Geometry check sheet. Reference: the model listing, model coordinates, mm. A direction names the side the tool comes from. Give positions to 0.01 mm unless a question says otherwise; leave off trailing zeros. Order: outer loops, then holes, each group sorted by start corner. A loop starts at its lowest first (then second) coordinate and runs counter-clockwise, first axis right, second up.
from build123d import *

# Parameters (mm, degrees)
SKETCH1_W           = 130
SKETCH1_H           = 64
SKETCH1_R           = 2.9575
BOSS_EXTRUDE1_DEPTH = 10
SKETCH2_W           = 130
SKETCH2_H           = 16
SKETCH2_R           = 2.75
BOSS_EXTRUDE2_DEPTH = 10
SKETCH3_W           = 160
SKETCH3_H           = 70
SKETCH3_R           = 2.25
SKETCH3_R_2         = 5.25
BOSS_EXTRUDE3_DEPTH = 7
SKETCH4_R           = 12
CUT_EXTRUDE1_DEPTH  = 3
FILLET1_R           = 5
CUT_EXTRUDE2_REACH  = 126.282
SKETCH5_R           = 2.9575
FILLET2_R           = 5
FILLET3_R           = 5


with BuildPart() as part:
    # Sketch1 → Boss-Extrude1 (new body)
    with BuildSketch(Plane.XY):
        Rectangle(SKETCH1_W, SKETCH1_H)
        with Locations((57, 16)):
            Circle(SKETCH1_R, mode=Mode.SUBTRACT)
        with Locations((57, -16)):
            Circle(SKETCH1_R, mode=Mode.SUBTRACT)
        with Locations((-57, -16)):
            Circle(SKETCH1_R, mode=Mode.SUBTRACT)
        with Locations((-57, 16)):
            Circle(SKETCH1_R, mode=Mode.SUBTRACT)
    extrude(amount=BOSS_EXTRUDE1_DEPTH)

    # Sketch2 → Boss-Extrude2 (add)
    with BuildSketch(Plane.XZ.offset(32)):
        with Locations((0, -8)):
            Rectangle(SKETCH2_W, SKETCH2_H)
        with Locations(Location((-40, -9, 0), (0, 0, 270))):
            Circle(SKETCH2_R, mode=Mode.SUBTRACT)
        with Locations(Location((40, -9, 0), (0, 0, 90))):
            Circle(SKETCH2_R, mode=Mode.SUBTRACT)
    extrude(amount=-BOSS_EXTRUDE2_DEPTH)

    # Sketch3 → Boss-Extrude3 (add)
    with BuildSketch(Plane(origin=(0, 32, 0), x_dir=(1, 0, 0), z_dir=(0, 1, 0))):
        with Locations((-15, -35)):
            Rectangle(SKETCH3_W, SKETCH3_H)
        with Locations(Location((48, -12.95, 0), (0, 0, 270))):
            Circle(SKETCH3_R, mode=Mode.SUBTRACT)
        with Locations(Location((-4.1, -18.05, 0), (0, 0, 270))):
            Circle(SKETCH3_R, mode=Mode.SUBTRACT)
        with Locations(Location((-4.1, -45.95, 0), (0, 0, 270))):
            Circle(SKETCH3_R, mode=Mode.SUBTRACT)
        with Locations(Location((46.7, -61.15, 0), (0, 0, 270))):
            Circle(SKETCH3_R, mode=Mode.SUBTRACT)
        with Locations(Location((-80, -58, 0), (0, 0, 270))):
            Circle(SKETCH3_R_2, mode=Mode.SUBTRACT)
        with BuildLine():
            Line((-83.039736831, -30.6), (-76.960263169, -30.6))
            ThreePointArc((-76.960263169, -30.6), (-72, -38), (-76.960263169, -45.4))
            Line((-76.960263169, -45.4), (-83.039736831, -45.4))
            ThreePointArc((-83.039736831, -45.4), (-88, -38), (-83.039736831, -30.6))
        make_face(mode=Mode.SUBTRACT)
        with BuildLine():
            Line((-83.039736831, -7.6), (-76.960263169, -7.6))
            ThreePointArc((-76.960263169, -7.6), (-72, -15), (-76.960263169, -22.4))
            Line((-76.960263169, -22.4), (-83.039736831, -22.4))
            ThreePointArc((-83.039736831, -22.4), (-88, -15), (-83.039736831, -7.6))
        make_face(mode=Mode.SUBTRACT)
    extrude(amount=BOSS_EXTRUDE3_DEPTH)

    # Sketch4 → Cut-Extrude1 (cut)
    # profile 1 of 6: a face of its own
    with BuildSketch(Plane.XZ.offset(-32)):
        with Locations((-80, 38)):
            Circle(SKETCH4_R)
    # profile 2 of 6: a face of its own
    with BuildSketch(Plane.XZ.offset(-32)):
        with Locations((-80, 15)):
            Circle(SKETCH4_R)
        with BuildLine():
            Line((-76.960263169, 7.6), (-83.039736831, 7.6))
            ThreePointArc((-83.039736831, 7.6), (-88, 15), (-83.039736831, 22.4))
            Line((-83.039736831, 22.4), (-76.960263169, 22.4))
            ThreePointArc((-76.960263169, 22.4), (-72, 15), (-76.960263169, 7.6))
        make_face(mode=Mode.SUBTRACT)
    # profile 3 of 6: a face of its own
    with BuildSketch(Plane.XZ.offset(-32)):
        with Locations((-80, 15)):
            Circle(SKETCH4_R)
    # profile 4 of 6: a face of its own
    with BuildSketch(Plane.XZ.offset(-32)):
        with Locations((-80, 38)):
            Circle(SKETCH4_R)
        with BuildLine():
            Line((-76.960263169, 30.6), (-83.039736831, 30.6))
            ThreePointArc((-83.039736831, 30.6), (-88, 38), (-83.039736831, 45.4))
            Line((-83.039736831, 45.4), (-76.960263169, 45.4))
            ThreePointArc((-76.960263169, 45.4), (-72, 38), (-76.960263169, 30.6))
        make_face(mode=Mode.SUBTRACT)
    # profile 5 of 6: a face of its own
    with BuildSketch(Plane.XZ.offset(-32)):
        with Locations((-80, 38)):
            Circle(SKETCH4_R)
    # profile 6 of 6: a face of its own
    with BuildSketch(Plane.XZ.offset(-32)):
        with Locations((-80, 15)):
            Circle(SKETCH4_R)
    extrude(amount=-CUT_EXTRUDE1_DEPTH, mode=Mode.SUBTRACT)

    # Fillet1
    fillet1_edges = [part.edges().sort_by_distance(p)[0] for p in [
        (-83.4278273, 33.5, 26.5),
        (-76.5721727, 33.5, 26.5),
    ]]
    fillet(fillet1_edges, radius=FILLET1_R)

    # Sketch5 → Cut-Extrude2 (cut, up to next)
    with BuildSketch(Plane(origin=(0, 0, 0), x_dir=(-1, 0, 0), z_dir=(0, 0, -1)), mode=Mode.PRIVATE) as cut_extrude2_sk1:
        with Locations((-50, -2)):
            Circle(SKETCH5_R)
    cut_extrude2_tool1 = extrude(cut_extrude2_sk1.sketch, amount=-CUT_EXTRUDE2_REACH, mode=Mode.PRIVATE) & part.part
    # Sketch5 → Cut-Extrude2 (cut, up to next)
    with BuildSketch(Plane(origin=(0, 0, 0), x_dir=(-1, 0, 0), z_dir=(0, 0, -1)), mode=Mode.PRIVATE) as cut_extrude2_sk2:
        with Locations((50, -2)):
            Circle(SKETCH5_R)
    cut_extrude2_tool2 = extrude(cut_extrude2_sk2.sketch, amount=-CUT_EXTRUDE2_REACH, mode=Mode.PRIVATE) & part.part
    add(cut_extrude2_tool1.solids().sort_by_distance((50, -2, 0))[0], mode=Mode.SUBTRACT)
    add(cut_extrude2_tool2.solids().sort_by_distance((-50, -2, 0))[0], mode=Mode.SUBTRACT)

    # Fillet2
    fillet2_edges = [part.edges().sort_by_distance(p)[0] for p in [
        (-65, -27, -16),
    ]]
    fillet(fillet2_edges, radius=FILLET2_R)

    # Fillet3
    fillet3_edges = [part.edges().sort_by_distance(p)[0] for p in [
        (65, -27, -16),
    ]]
    fillet(fillet3_edges, radius=FILLET3_R)


solid = part.part
Item 1: Draft check along Y on faces 6 (the flat face through (-16, 32, 42)), 7 (the cylindrical face through (-79.769, 35.451, 52.755)), 8 (the cylindrical face through (-55.41, -13.506, 4.93)). Enter one of: released by +Y, released by -Y, zero draft, split by the parting line, or undercut.
Reported:
face 6: released by -Y
face 7: zero draft
face 8: undercut
Item 2: Sectioned sample at D-D (z = 38). Enter the section's corners in (x, y).
Reported:
outline: (-95, 32) - (-92, 32) - (-92, 35) - (-88, 35) - (-88, 39) - (-95, 39) - close; (-72, 35) - (-68, 35) - (-68, 32) - (65, 32) - (65, 39) - (-72, 39) - close
Item 3: Sectioned sample at C-C (y = -16). Enter the section's corners in (x, z).
Reported:
outline: (-65, 0) - (-59.96, 0) - (-59.96, 10) - (-65, 10) - close; (-54.04, 0) - (54.04, 0) - (54.04, 10) - (-54.04, 10) - close; (59.96, 0) - (65, 0) - (65, 10) - (59.96, 10) - close
Item 4: Gauge pin test, flat ends, axial feed: pin 1 (10 mm diameter, centred on x = -32, z = 52.5, fed in from -Y); pin 2 (3 mm diameter, centred on x = -79, y = 37, fed in from -Z); pin 3 (7 mm diameter, centred on x = 57, y = 16, fed in from +Z). Record the tip position at first contact, or that the pin passes through.
Reported:
pin 1: stops at y = 32
pin 2: stops at z = 0
pin 3: stops at z = 10
Item 5: Sectioned sample at B-B (x = -4.1). Enter the section's corners in (y, z), and give its area (3 significant figures).
Reported:
outline: (-32, -16) - (-22, -16) - (-22, 0) - (39, 0) - (39, 15.8) - (32, 15.8) - (32, 10) - (-32, 10) - close; (32, 20.3) - (39, 20.3) - (39, 43.7) - (32, 43.7) - close; (32, 48.2) - (39, 48.2) - (39, 70) - (32, 70) - close
area: 1,230 mm2
Item 6: Sectioned sample at A-A (z = 61.15). Enter the section's corners in (x, y), and give its area (3 significant figures).
Reported:
outline: (-95, 32) - (-84.2, 32) - (-84.2, 39) - (-95, 39) - close; (-75.8, 32) - (44.45, 32) - (44.45, 39) - (-75.8, 39) - close; (48.95, 32) - (65, 32) - (65, 39) - (48.95, 39) - close
area: 1,030 mm2
Item 7: Scan lines: L1, parallel to X at y = -27.75, z = -9; L2, parallel to Z at x = 40, y = -27; L3, parallel to Y at x = -57, z = 4. Record each from-to range of solid material in increasing order.
Reported:
L1: x = -65 to -42.75, -37.25 to 37.25, 42.75 to 65
L2: z = -16 to -11.75, -6.25 to 10
L3: y = -32 to -18.96, -13.04 to 13.04, 18.96 to 39
Item 8: Set-up check for faces 1 (the flat face through (65, 11, 9)), 2 (the flat face through (-1, -32, -3)), 3 (the cylindrical face through (-80, 33, 3)), 4 (the flat face through (-1, 0, 10)), 5 (the flat face through (-80, 37, 30.6)): record each of +Z, -Z, +X, -X, +Y, -Y from which the full face is reachable in a straight line by a thin tool's end or side.
Reported:
face 1: +Z, -Z, +X, +Y, -Y
face 2: +Z, -Z, +X, -X, -Y
face 3: -Y
face 4: +Z, +X, -X, -Y
face 5: +Y, -Y
